Part model, mm, in its own coordinate system. Give positions to 0.01 mm unless a question says otherwise; leave off trailing zeros. Loops run counter-clockwise (first coordinate to the right, second up) from the corner with the lowest first, then second, coordinate; pieces in that order, holes last. Notation, with made-up numbers: M 62.25,71.5 L 97.25,71.5 A22 ccw 97.25,78.5 Z; hole C -9.5,34 d3. An arc over 180 degrees is marked long. Answer in a Markdown table with one row per item.
from build123d import *

# Parameters (mm, degrees)
F1_DEPTH = 10
F2_W     = 5
F2_H     = 5
F3_DEPTH = 5
F4_W     = 5
F4_H     = 5
F5_DEPTH = 2
F6_SIZE  = 1


with BuildPart() as f1:
    # F0 (on Front) → F1 (new body)
    with BuildSketch(Plane.XZ):
        Polygon((21.76041, -48.874682), (0, 0), (0, -49.2), (6.8, -49.2), (6.718023, -31.700192), (14.426186, -49.013011), align=None)
    extrude(amount=F1_DEPTH)

    # F2 (on face) → F3 (cut)
    with BuildSketch(Plane(origin=(0, 0, -49.2), x_dir=(1, 0, 0), z_dir=(0, 0, -1))):
        with Locations((3.4, 5)):
            Rectangle(F2_W, F2_H)
    extrude(amount=-F3_DEPTH, mode=Mode.SUBTRACT)

    # F4 (on face) → F5 (cut)
    with BuildSketch(Plane(origin=(0.929221, 0, -49.267573), x_dir=(0.999822, 0, 0.018857), z_dir=(0.018857, 0, -0.999822))):
        with Locations((17.16713, 5)):
            Rectangle(F4_W, F4_H)
    extrude(amount=-F5_DEPTH, mode=Mode.SUBTRACT)

    # F6
    f6_edges = [f1.edges().sort_by_distance(p)[0] for p in [
        (10.880205, -10, -24.437341),
        (10.572105, -10, -40.356601),
        (6.759011, 0, -40.450096),
        (6.759011, -10, -40.450096),
        (0, -10, -24.6),
        (0, 0, -24.6),
        (10.572105, 0, -40.356601),
        (10.880205, 0, -24.437341),
    ]]
    chamfer(f6_edges, length=F6_SIZE)


solid = f1.part
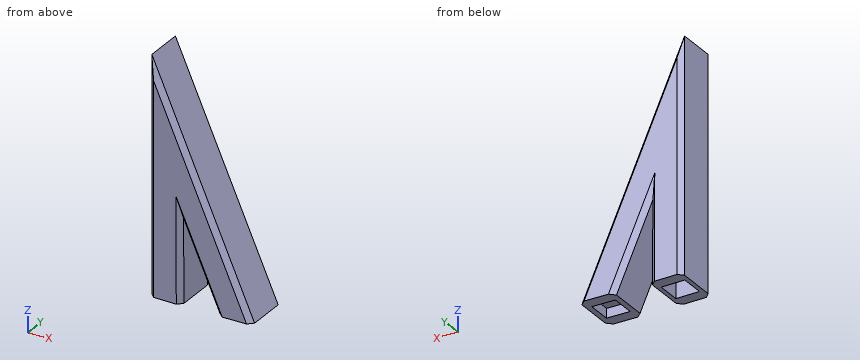
(1) Saw through at D-D (z = -8). Write the cut outline in (x, y).
Recorded:
| item | result |
|---|---|
| outline | M 0,-9 L 1,-10 L 2.47,-10 L 3.56,-9 L 3.56,-1 L 2.47,0 L 1,0 L 0,-1 Z |
(2) Saw through at B-B (z = -42.5). Write the cut outline in (x, y), plus the area to 3 significant figures.
Recorded:
| item | result |
|---|---|
| outline | M 0,-9 L 1,-10 L 5.77,-10 L 6.77,-9 L 6.77,-1 L 5.77,0 L 1,0 L 0,-1 Z; M 11.53,-9 L 12.62,-10 L 17.83,-10 L 18.92,-9 L 18.92,-1 L 17.83,0 L 12.62,0 L 11.53,-1 Z |
| area | 137 mm^2 |
(3) Drill centre lines: line 1 along X through (y, z) = (-6.25, -33.5); line 2 along X through (y, z) = (-8, -39); line 3 along Z through (x, y) = (11.25, -7.5). Where is each one in solid material? Low to high.
Recorded:
| item | result |
|---|---|
| line 1 | x = 0 to 6.73, 7.52 to 14.92 |
| line 2 | x = 0 to 6.75, 9.97 to 17.36 |
| line 3 | z = -41.88 to -25.27 |
(4) Pin check, flat tips, straight feed: pin 1 Ø4 at (x, y) = (8.5, -1.5) entering from +Z; pin 2 Ø5.5 at (y, z) = (-4, -47) entering from +X; pin 3 Ø1 at (x, y) = (12, -3) entering from -Z; pin 4 Ø2.5 at (x, y) = (3.5, -4) entering from -Z. Stop position of each tip, or through.
Recorded:
| item | result |
|---|---|
| pin 1 | stops at z = -14.6 |
| pin 2 | stops at x = 21.76 |
| pin 3 | stops at z = -44.69 |
| pin 4 | stops at z = -44.2 |
(5) Saw through at C-C (x = 7.75). Write the cut outline in (y, z), plus the area to 3 significant figures.
Recorded:
| item | result |
|---|---|
| outline | M -10,-31.56 L -9,-34.02 L -1,-34.02 L 0,-31.56 L 0,-19.87 L -1,-17.41 L -9,-17.41 L -10,-19.87 Z |
| area | 161 mm^2 |
(6) Saw through at A-A (y = -6). Write the cut outline in (x, z), plus the area to 3 significant figures.
Recorded:
| item | result |
|---|---|
| outline | M 0,-49.2 L 0.9,-49.2 L 0.9,-44.2 L 5.9,-44.2 L 5.9,-49.2 L 6.8,-49.2 L 6.72,-31.7 L 14.43,-49.01 L 15.59,-48.99 L 15.56,-46.99 L 20.56,-46.9 L 20.59,-48.9 L 21.76,-48.87 L 0,0 Z |
| area | 435 mm^2 |
